Check sheet for the modelled part. Datum: model origin and axes. Units: mm. Face numbers are marked on the shaded views. A direction names the side the tool comes from. Round coordinates to 2 decimals unless told otherwise and drop trailing zeros. Write each loop counter-clockwise with the first axis right and the second up, starting at its lowest first coordinate (ties: lowest second). Pieces come first, ordered by that corner, then holes. Notation, with made-up numbers: (55.25, 65) -> (82.25, 65) arc R24 cw to (82.25, 76) -> close; hole circle Ø1 at (51.25, 85.5). An arc over 180 degrees is marked (long way). One line per item, written item: value.
Solid Edge part; units mm, degrees
sketch "Sketch1" plane through (0, 0, 0) normal (1, 0, 0) x (0, 1, 0)
  arc A0 (0, 0) -> (-30, -30) centre (0, -30) ccw
  line L0 (-30, -40) -> (-30, -30)
  line L1 (-10, -40) -> (-30, -40)
  line L2 (-10, -30) -> (-10, -40)
  arc A1 (0, -20) -> (-10, -30) centre (0, -30) ccw
  line L3 (10, -20) -> (0, -20)
  line L4 (10, 0) -> (10, -20)
  line L5 (0, 0) -> (10, 0)
extrude "Protrusion1" add sketch "Sketch1" against normal blind 12
sketch "Sketch2" plane through (0, 0, 0) normal (0, 0, 1) x (1, 0, 0)
  line L0 (0, 10) -> (-12, 10)
  arc A0 (-12, 10) -> (0, 10) centre (-6, 24.8324) cw
  circle A1 centre (-6, 24.8324) radius 8
extrude "ExtrudedProtrusion_3" add sketch "Sketch2" against normal blind 20
sketch "Sketch3" plane through (-6, -20, -40) normal (0, 0, -1) x (-1, 0, 0)
  line L0 (-26, 60) -> (26, 60)
  line L1 (26, 60) -> (26, -15)
  line L2 (26, -15) -> (0, -15)
  line L3 (0, -15) -> (-26, -15)
  line L4 (-26, -15) -> (-26, -5)
  line L5 (-26, -5) -> (-26, 50)
  line L6 (-26, 50) -> (-26, 60)
extrude "ExtrudedProtrusion_4" add sketch "Sketch3" along normal blind 15
sketch "Sketch4" plane through (-6, -20, -40) normal (0, 0, -1) x (-1, 0, 0)
  circle A0 centre (16, 55) radius 2.5
  circle A1 centre (-16, 55) radius 2.5
  circle A2 centre (-16, -10) radius 2.5
  circle A3 centre (16, -10) radius 2.5
extrude "ExtrudedCutout_1" cut sketch "Sketch4" along normal blind 15
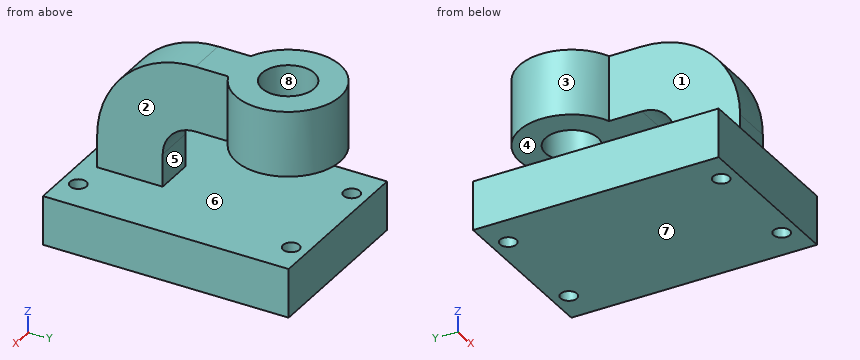
Item 1: Sectioned sample at D-D (x = -13). Enter the section's corners in (y, z).
Result set:
outline: (-35, -55) -> (40, -55) -> (40, -40) -> (-35, -40) -> close; (10.44, -20) -> (20.96, -20) -> (20.96, 0) -> (10.44, 0) -> close; (28.71, -20) -> (39.22, -20) -> (39.22, 0) -> (28.71, 0) -> close
Item 2: Sectioned sample at B-B (x = -6). Enter the section's corners in (y, z).
Result set:
outline: (-35, -55) -> (40, -55) -> (40, -40) -> (-10, -40) -> (-10, -30) arc R10 cw to (0, -20) -> (16.83, -20) -> (16.83, 0) -> (0, 0) arc R30 ccw to (-30, -30) -> (-30, -40) -> (-35, -40) -> close; (32.83, -20) -> (40.83, -20) -> (40.83, 0) -> (32.83, 0) -> close
Item 3: Depth check by flat-ended pin: pin 1 (1 mm diameter, centred on x = 8, z = -22, fed in from +Y); pin 2 (8 mm diameter, centred on x = -6, z = -35.5, fed in from +Y); pin 3 (1.5 mm diameter, centred on x = 1.5, y = -23, fed in from +Z); pin 4 (1 mm diameter, centred on y = -20.5, z = -21.5, fed in from +X). Enter the tip coordinate at first touch or a pass-through.
Result set:
pin 1: through
pin 2: y = -10
pin 3: z = -40
pin 4: x = 0
Item 4: Sectioned sample at C-C (y = 35). Enter the section's corners in (x, z).
Result set:
outline: (-32, -55) -> (-24.5, -55) -> (-24.5, -40) -> (-32, -40) -> close; (-19.5, -55) -> (7.5, -55) -> (7.5, -40) -> (-19.5, -40) -> close; (-18.35, -20) -> (6.35, -20) -> (6.35, 0) -> (-18.35, 0) -> close; (12.5, -55) -> (20, -55) -> (20, -40) -> (12.5, -40) -> close
Item 5: Material ranges on line 1 along Y through (x, z) = (10, -51); line 2 along X through (y, z) = (-8.5, -17.5); line 3 along Y through (x, z) = (-6, -5), recorded low to high.
Result set:
line 1: -35 to -32.5, -27.5 to 32.5, 37.5 to 40
line 2: -12 to 0
line 3: -16.58 to 16.83, 32.83 to 40.83
Item 6: Tool access check on the marked faces 1, 2, 3 and 4. Record the directions out of +Z, -Z, +X, -X, +Y, -Y that give a thin tool (end or side, any length) a straight path to the whole face; none if there is none.
Result set:
face 1: +Z, -X, -Y
face 2: +Z, +X, -Y
face 3: +Z
face 4: +X, -X, +Y
Item 7: Sectioned sample at A-A (z = -46). Enter the section's corners in (x, y), then the cut area to 3 significant figures.
Result set:
outline: (-32, -35) -> (20, -35) -> (20, 40) -> (-32, 40) -> close; hole circle Ø5 at (-22, -30); hole circle Ø5 at (-22, 35); hole circle Ø5 at (10, -30); hole circle Ø5 at (10, 35)
area: 3,820 mm^2
Item 8: Release check for a two-part mould opening along Z. For the marked faces 5, 6, 7 and 8 record: pulls with the +Z half, pulls with the -Z half, needs draft (parallel to the pull), parting line crosses it, or undercut.
Result set:
face 5: undercut
face 6: undercut
face 7: pulls with the -Z half
face 8: needs draft
